Source: three-view drawing plus pictorial views. Frame: mm from the lowest corner of the part. Give positions to 0.01 mm unless a question says otherwise; leave off trailing zeros. Order: outer loops, then holes, each group sorted by start corner. A loop starts at its lowest first (then second) coordinate and runs counter-clockwise, first axis right, second up. Notation, with made-up numbers: (46, 36) -> (56, 36) arc R33 ccw to (56, 72) -> close; hole circle Ø4 at (40.5, -4). An arc over 180 degrees is marked (long way). Answer in a Markdown table with one row per item.
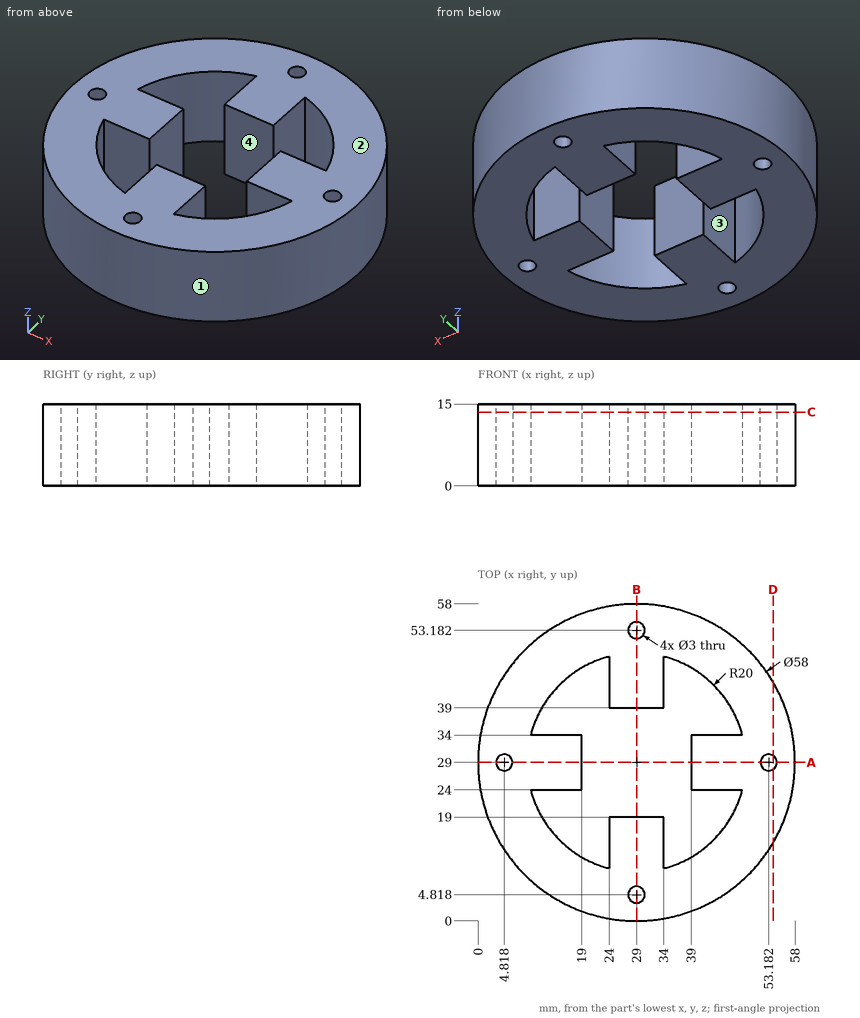
(1) Pull-direction query (X, two-part tool) for the marked faces 1, 2, 3 and 4; classes: +X half, -X half, draft (parallel to the pull), parting line (faces both ways), or undercut.
A:
| item | result |
|---|---|
| face 1 | parting line |
| face 2 | draft |
| face 3 | undercut |
| face 4 | undercut |
(2) First-contact query: pin 1 Ø5 at (x, z) = (19, 3.5) entering from -Y; pin 2 Ø4.5 at (y, z) = (14.5, 11) entering from +X (1 decimal); pin 3 Ø5 at (x, z) = (7.5, 11.5) entering from +Y. Flat tips, straight axial feed; report the tip coordinate or a pass-through.
A:
| item | result |
|---|---|
| pin 1 | stops at y = 0.99 |
| pin 2 | stops at x = 55.3 |
| pin 3 | stops at y = 50.91 |
(3) Section query C-C (z = 13.5). Return the cut outline in (x, y) (1 decimal).
A:
| item | result |
|---|---|
| outline | circle Ø58 at (29, 29); hole circle Ø3 at (4.8, 29); hole (9.6, 24) arc R20 ccw to (24, 9.6) -> (24, 19) -> (34, 19) -> (34, 9.6) arc R20 ccw to (48.4, 24) -> (39, 24) -> (39, 34) -> (48.4, 34) arc R20 ccw to (34, 48.4) -> (34, 39) -> (24, 39) -> (24, 48.4) arc R20 ccw to (9.6, 34) -> (19, 34) -> (19, 24) -> close; hole circle Ø3 at (29, 4.8); hole circle Ø3 at (29, 53.2); hole circle Ø3 at (53.2, 29) |
(4) Section query A-A (y = 29). Return the cut outline in (x, z), plus the area to 3 significant figures.
A:
| item | result |
|---|---|
| outline | (0, 0) -> (3.32, 0) -> (3.32, 15) -> (0, 15) -> close; (6.32, 0) -> (19, 0) -> (19, 15) -> (6.32, 15) -> close; (39, 0) -> (51.68, 0) -> (51.68, 15) -> (39, 15) -> close; (54.68, 0) -> (58, 0) -> (58, 15) -> (54.68, 15) -> close |
| area | 480 mm^2 |
(5) Section query D-D (x = 54). Return the cut outline in (y, z).
A:
| item | result |
|---|---|
| outline | (14.3, 0) -> (27.74, 0) -> (27.74, 15) -> (14.3, 15) -> close; (30.26, 0) -> (43.7, 0) -> (43.7, 15) -> (30.26, 15) -> close |
(6) Ray query, probe 1 along Y at (x, z) = (29, 7.5); probe 2 along Y at (x, z) = (47, 11.25) (1 decimal); probe 3 along X at (y, z) = (40, 1.25) (1 decimal). Return the intervals inside material, ascending.
A:
| item | result |
|---|---|
| probe 1 | y = 0 to 3.32, 6.32 to 19, 39 to 51.68, 54.68 to 58 |
| probe 2 | y = 6.3 to 20.3, 24 to 34, 37.7 to 51.7 |
| probe 3 | x = 2.2 to 12.3, 24 to 34, 45.7 to 55.8 |
